from build123d import *

# Parameters (mm, degrees)
SKETCH1_R           = 4.953
SKETCH1_W           = 3.175
SKETCH1_H           = 9.525
BOSS_EXTRUDE1_DEPTH = 3.175


with BuildPart() as part:
    # Sketch1 → Boss-Extrude1 (new body)
    with BuildSketch(Plane.XY):
        with BuildLine():
            Line((-25.372181386, 1.188449288), (-15.875, 203.943595206))
            ThreePointArc((-15.875, 203.943595206), (0, 219.092405697), (15.875, 203.943595206))
            Line((15.875, 203.943595206), (25.372181386, 1.188449288))
            ThreePointArc((25.372181386, 1.188449288), (0, -25.4), (-25.372181386, 1.188449288))
        make_face()
        Circle(SKETCH1_R, mode=Mode.SUBTRACT)
        Polygon((-6.35, 200.025), (6.35, 200.025), (6.35, 196.85), (9.525, 196.85), (9.525, 184.15), (6.35, 184.15), (6.35, 180.975), (-6.35, 180.975), (-6.35, 184.15), (-9.525, 184.15), (-9.525, 196.85), (-6.35, 196.85), align=None, mode=Mode.SUBTRACT)
        with Locations((-17.9197, 30.1625)):
            Rectangle(SKETCH1_W, SKETCH1_H, mode=Mode.SUBTRACT)
        with Locations((0, 152.4)):
            Rectangle(SKETCH1_W, SKETCH1_H, mode=Mode.SUBTRACT)
        with Locations((17.9197, 30.1625)):
            Rectangle(SKETCH1_W, SKETCH1_H, mode=Mode.SUBTRACT)
    extrude(amount=BOSS_EXTRUDE1_DEPTH)


solid = part.part
The model under review builds one solid part; all positions refer to its coordinate system, in mm. Round coordinates to 2 decimals unless told otherwise and drop trailing zeros. Order: outer loops, then holes, each group sorted by start corner. A loop starts at its lowest first (then second) coordinate and runs counter-clockwise, first axis right, second up. Notation, with made-up numbers: (45.25, 81.25) -> (50.25, 81.25) arc R21 ccw to (50.25, 98.25) -> close; hole circle Ø11 at (6.5, 70.5). An arc over 180 degrees is marked (long way). Write item = value, one per line. Start each with the question number.
Item 1: Consider section A-A on z = 1.2. Count the separate pieces of the cut face and the enclosed holes in it, plus the area to 3 significant figures.
Item 2: Clearance check with flat-ended pins moving along their axes: pin 1 Ø1.6 at (y, z) = (192, 2.5) entering from -X; pin 2 Ø1 at (y, z) = (187.5, 1.5) entering from +X; pin 3 Ø1 at (y, z) = (152, 2.5) entering from +X. State where each tip first meets the part, or that it passes through.
Item 3: For line 1 along X through (y, z) = (28.5, 2.2); line 2 along Y through (x, z) = (-3.5, 2.85) (3 decimals); line 3 along X through (y, z) = (31, 0.55), list the stretches that pass through material, from the lowest coordinate up.
Item 4: Consider section B-B on y = 19. Write out the cut boundary in (x, z) (3 decimals).
Item 5: Mouldability with a two-part tool opening along Y and no side actions: class faces 1 (the face through (0, 99, 0)), 2 (the face through (-20.69, 101.15, 1.57)), 3 (the face through (-0.64, 4.91, 1.57)) as released by +Y, released by -Y, zero draft, split by the parting line, or undercut.
Conclusion:
q1.separate_pieces = 1
q1.enclosed_holes = 5
q1.area = 9,320 mm2
q2.pin_1 = -16.47
q2.pin_2 = 16.67
q2.pin_3 = 18.33
q3.line_1 = -24.09 to -19.51, -16.33 to 16.33, 19.51 to 24.09
q3.line_2 = -25.158 to -3.505, 3.505 to 180.975, 200.025 to 218.702
q3.line_3 = -23.98 to -19.51, -16.33 to 16.33, 19.51 to 23.98
q4.outline = (-24.538, 0) -> (24.538, 0) -> (24.538, 3.175) -> (-24.538, 3.175) -> close
q5.face_1 = zero draft
q5.face_2 = released by +Y
q5.face_3 = undercut
